Geometry check sheet. Reference: the model listing, model coordinates, mm. A direction names the side the tool comes from. Round coordinates to 2 decimals unless told otherwise and drop trailing zeros. Order: outer loops, then holes, each group sorted by start corner. A loop starts at its lowest first (then second) coordinate and runs counter-clockwise, first axis right, second up. Notation, with made-up numbers: (-23.5, 86) -> (-9.5, 86) arc R8 cw to (-9.5, 91) -> close; hole circle Ø9 at (-3.5, -39). An arc over 180 degrees is marked (long way). Use a Markdown table: item, result. Add a question column.
Item 1: Sectioned sample at C-C, the plane z = 106. Record the cut outline in (x, y).
Item 2: Material ranges on probe 1 along Y at (x, z) = (7, 603), recorded low to high. Write a range as [from, to].
Item 3: Sectioned sample at A-A, the plane x = 4.75. Record the cut outline in (y, z).
Item 4: Mould release check, pull along X, two halves, no side actions. Record for faces 3 (the flat face through (7, 1, 375)), 4 (the flat face through (15, 7, 365)), 5 (the flat face through (1, 8, 375)), 6 (the flat face through (0.7, 7.6, 0)): pulls with the +X half, pulls with the -X half, needs draft (parallel to the pull), parting line crosses it, or undercut.
Item 5: Set-up check for faces 1 (the flat face through (7, 0, 365)), 2 (the flat face through (14, 7, 375)): record each of +Z, -Z, +X, -X, +Y, -Y from which the full face is reachable in a straight line by a thin tool's end or side.
Autodesk Inventor part; units mm, degrees
ref_plane "YZ Plane" through (0, 0, 0) normal (1, 0, 0) x (0, 1, 0)
ref_plane "XZ Plane" through (0, 0, 0) normal (0, 1, 0) x (-1, 0, 0)
ref_plane "XY Plane" through (0, 0, 0) normal (0, 0, 1) x (1, 0, 0)
sketch "スケッチ1" plane through (0, 0, 0) normal (0, 0, 1) x (1, 0, 0)
  line L0 (0, 0) -> (15, 0)
  line L1 (15, 0) -> (15, 15)
  line L2 (15, 15) -> (0, 15)
  line L3 (0, 15) -> (0, 0)
  dimension "d0" = 15
  dimension "d1" = 15
extrude "押し出し1" add sketch "スケッチ1" along normal blind 740
sketch "スケッチ2" plane through (0, 0, 0) normal (0, 0, -1) x (-1, 0, 0)
  point P0 (0, 0)
sketch "スケッチ3" plane through (0, 0, 740) normal (0, 0, 1) x (1, 0, 0)
  line L0 (1, 1) -> (14, 1)
  line L1 (14, 1) -> (14, 14)
  line L2 (14, 14) -> (1, 14)
  line L3 (1, 14) -> (1, 1)
  line L4 (0, 15) -> (0, 0)
  line L5 (0, 0) -> (15, 0)
  dimension "d4" = 13
  dimension "d5" = 13
  dimension "d6" = 1
  dimension "d7" = 1
extrude "押し出し2" cut sketch "スケッチ3" against normal blind 740
equation "\"BendRadius\" = Thickness"
equation "\"BendReliefWidth\" = Thickness"
equation "\"BendReliefDepth\" = 0.5 * Thickness"
equation "\"CornerReliefSize\" = 4 * Thickness"
equation "\"MinimumRemnant\" = 2 * Thickness"
equation "\"TransitionRadius\" = BendRadius"
equation "\"JacobiRadiusSize\" = BendRadius"
equation "\"GapSize\" = Thickness"
properties part number "足3"
Found:
| question | item | result |
|---|---|---|
| 1 | outline | (0, 0) -> (15, 0) -> (15, 15) -> (0, 15) -> close; hole (1, 1) -> (14, 1) -> (14, 14) -> (1, 14) -> close |
| 2 | probe 1 | y = [0, 1], [14, 15] |
| 3 | outline | (0, 0) -> (1, 0) -> (1, 740) -> (0, 740) -> close; (14, 0) -> (15, 0) -> (15, 740) -> (14, 740) -> close |
| 4 | face 3 | undercut |
| 4 | face 4 | pulls with the +X half |
| 4 | face 5 | undercut |
| 4 | face 6 | needs draft |
| 5 | face 1 | +Z, -Z, +X, -X, -Y |
| 5 | face 2 | +Z, -Z |
